from build123d import *

# Parameters (mm, degrees)
SKETCH1_R               = 9.525
BOSS_EXTRUDE1_DEPTH     = 304.8
SKETCH3_W               = 23.44415324
SKETCH3_H               = 6.388604027
CUT_EXTRUDE1_DEPTH      = 158.75
CUT_EXTRUDE2_DEPTH      = 306.097511052
CUT_EXTRUDE2_DEPTH_BACK = 306.097511052
SKETCH8_R               = 2.54


with BuildPart() as part:
    # Sketch1 → Boss-Extrude1 (new body)
    with BuildSketch(Plane.XY):
        Circle(SKETCH1_R)
    extrude(amount=-BOSS_EXTRUDE1_DEPTH)

    # Sketch3 → Cut-Extrude1 (cut)
    with BuildSketch(Plane.XY):
        with Locations((0.072269276, 11.131802014)):
            Rectangle(SKETCH3_W, SKETCH3_H)
    extrude(amount=-CUT_EXTRUDE1_DEPTH, mode=Mode.SUBTRACT)

    # Sketch8 → Cut-Extrude2 (cut, two sides: drawn at the far end of the back side and taken through both)
    with BuildSketch(Plane(origin=(0, 0, 0), x_dir=(0, 0, -1), z_dir=(1, 0, 0)).offset(-CUT_EXTRUDE2_DEPTH_BACK)):
        with Locations((238.125, 0)):
            Circle(SKETCH8_R)
    extrude(amount=CUT_EXTRUDE2_DEPTH + CUT_EXTRUDE2_DEPTH_BACK, mode=Mode.SUBTRACT)


solid = part.part
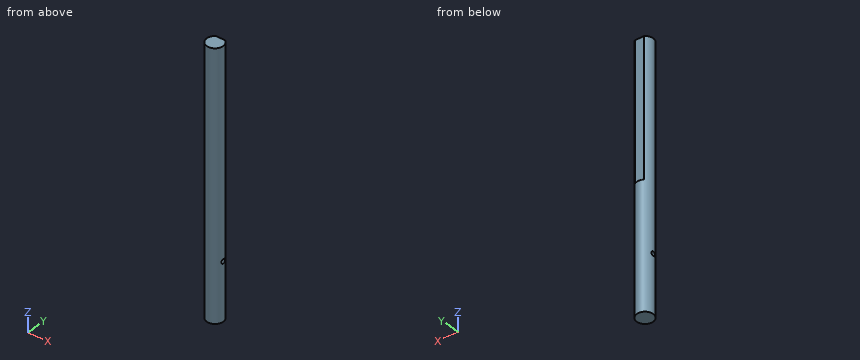
Here's how the part is built. I have some questions about the finished solid (model axes, mm). Give positions to 0.01 mm unless a question says otherwise; leave off trailing zeros. Order: outer loops, then holes, each group sorted by start corner. A loop starts at its lowest first (then second) coordinate and runs counter-clockwise, first axis right, second up. Notation, with made-up numbers: M -21,61.25 L 16,61.25 A20 ccw 16,73.25 Z; hole C -4.75,74 d2. An arc over 180 degrees is marked long. Answer as a JSON object with one key per item and string values. Group by question number.
1) I'm going to push flat-ended pins straight in: pin 1 Ø0.8 at (x, y) = (0, 9) entering from +Z; pin 2 Ø2 at (y, z) = (-4.5, -113.5) entering from +X; pin 3 Ø5.5 at (x, z) = (1, -86) entering from +Y; pin 4 Ø3 at (y, z) = (0, -238.125) entering from +X. Where does each tip first touch, or does it pass through?
2) Please list where these lines run through material, in increasing order: L1, parallel to Z at x = 4.25, y = -0.5; L2, parallel to Z at x = 8, y = 0 (3 decimals); L3, parallel to Z at x = -2.75, y = 8. Write a range as [from, to].
3) Suppose I cut it at D-D, the plane z = -279. Write out the boundary of the cut face in (x, y) (3 decimals).
4) Suppose I cut it at A-A, the plane y = 0. Write out the boundary of the cut face in (x, z) (3 decimals), plus the area to 3 significant figures.
Results found:
{
 "1": {"pin 1": "z = -158.75", "pin 2": "x = 8.86", "pin 3": "y = 7.94", "pin 4": "through"},
 "2": {"L1": "[-304.8, -240.62], [-235.63, 0]", "L2": "[-304.8, -240.665], [-235.585, 0]", "L3": "[-304.8, -158.75]"},
 "3": {"outline": "C 0,0 d19.05"},
 "4": {"outline": "M -9.525,-304.8 L 9.525,-304.8 L 9.525,-240.665 L -9.525,-240.665 Z; M -9.525,-235.585 L 9.525,-235.585 L 9.525,0 L -9.525,0 Z", "area": "5,710 mm²"}
}
